from build123d import *

# Parameters (mm, degrees)
F1_DEPTH  = 6
F2_W      = 104
F2_H      = 80
F2_W_2    = 6
F3_DEPTH  = 6
F5_DEPTH  = 104
F7_DEPTH  = 200
F8_R      = 11.4401294272
F10_DEPTH = 200
F11_W     = 86
F11_H     = 24.3039056659
F12_DEPTH = 1
F13_W     = 32.8389904462
F13_H     = 60.4005604982
F14_DEPTH = 1


with BuildPart() as f1:
    # F0 (on Front) → F1 (new body)
    with BuildSketch(Plane.XZ):
        Polygon((-88, 80), (-80, 37.097658962), (-80, 80), align=None)
        Polygon((-80, 0), (0, 0), (0, 80), (-80, 80), (-80, 37.097658962), align=None)
    extrude(amount=F1_DEPTH)

    # F2 (on face) → F3 (join)
    with BuildSketch(Plane.YZ):
        with Locations((52, 40)):
            Rectangle(F2_W, F2_H)
        with Locations((-3, 40)):
            Rectangle(F2_W_2, F2_H)
    extrude(amount=F3_DEPTH)

    # F5 (add, through all): a face of the model
    f5_faces = [f1.faces().sort_by_distance(p)[0] for p in [
        (-41.1141866674, 0, 40.6711029977),
    ]]
    extrude(f5_faces, amount=F5_DEPTH)

    # F6 (on face) → F7 (cut)
    with BuildSketch(Plane.YZ.offset(6)):
        Polygon((104, 0), (49, 10.5), (-6, 0), align=None)
    extrude(amount=-F7_DEPTH, mode=Mode.SUBTRACT)

    # F8 (on face) → F10 (cut)
    with BuildSketch(Plane(origin=(0, 104, 0), x_dir=(-1, 0, 0), z_dir=(0, 1, 0))):
        with Locations((58.3457089961, 57.7158816159)):
            Circle(F8_R)
    extrude(amount=-F10_DEPTH, mode=Mode.SUBTRACT)

    # F11 (on face) → F12 (join)
    with BuildSketch(Plane(origin=(-70.6266357892, 0, -13.1697495438), x_dir=(0, -1, 0), z_dir=(-0.983055103, 0, -0.1833102957))):
        with Locations((-49, 72.5469328463)):
            Rectangle(F11_W, F11_H)
    extrude(amount=F12_DEPTH)

    # F13 (on face) → F14 (join)
    with BuildSketch(Plane(origin=(0, 104, 0), x_dir=(-1, 0, 0), z_dir=(0, 1, 0))):
        with Locations((20.5245364923, 30.2002802491)):
            Rectangle(F13_W, F13_H)
    extrude(amount=F14_DEPTH)


solid = f1.part
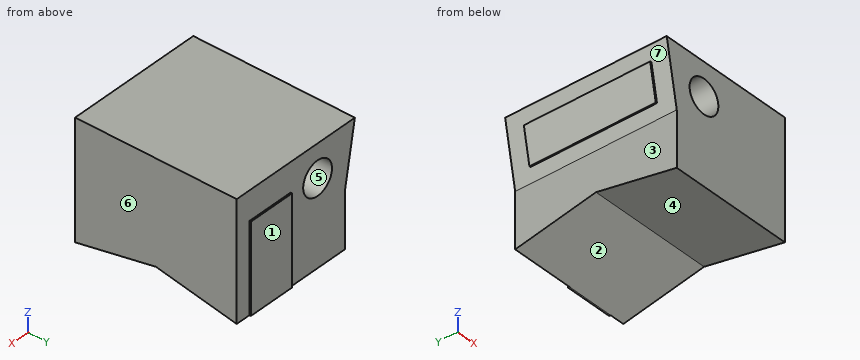
Geometry: final body of the model. Coordinates: model frame, mm. Face numbers are marked on the shaded views. A direction names the side the tool comes from. Give positions to 0.01 mm unless a question says otherwise; leave off trailing zeros. Loops run counter-clockwise (first coordinate to the right, second up) from the corner with the lowest first, then second, coordinate; pieces in that order, holes last. Notation, with made-up numbers: (-40, 30.5) -> (-9, 30.5) arc R22 ccw to (-9, 56.5) -> close; hole circle Ø5 at (-26.75, -20). An arc over 180 degrees is marked (long way). Put each result on its own line as item: value.
1. Pin query (flat end, axial travel): P1, Ø2.5, axis at x = -85.5, z = 59.5, coming from the +Y side; P2, Ø0.8, axis at y = 104.5, z = 15.5, coming from the -X side; P3, Ø6, axis at x = -66.5, z = 29.5, coming from the +Y side; P4, Ø13.5, axis at x = -58.35, z = 57.72, coming from the -Y side. Return the tip coordinate at first contact, or that it passes through.
Taken from the geometry:
P1: stops at y = 92
P2: stops at x = -36.94
P3: stops at y = 104
P4: passes through
2. Set-up query: the marked faces 1, 2 and 3. Return all of +Z, -Z, +X, -X, +Y, -Y with unobstructed straight access to the full face (end or side cutting, diameter ignored); none if empty.
Taken from the geometry:
face 1: +Z, -Z, +X, -X, +Y
face 2: -Z, +X, -X
face 3: -Z, -X, +Y, -Y
3. Cut plane A-A (z = 8.5). Return the cut outline in (x, y).
Taken from the geometry:
outline: (-80, -6) -> (6, -6) -> (6, 38.52) -> (-80, 38.52) -> close; (-80, 59.48) -> (6, 59.48) -> (6, 104) -> (-4.11, 104) -> (-4.11, 105) -> (-36.94, 105) -> (-36.94, 104) -> (-80, 104) -> close
4. Pull-direction query (Z, two-part tool) for the marked faces 4, 5, 6 and 7; classes: released by +Z, released by -Z, zero draft, split by the parting line, or undercut.
Taken from the geometry:
face 4: released by -Z
face 5: undercut
face 6: zero draft
face 7: undercut
5. Cut plane D-D (x = -28). Return the cut outline in (y, z).
Taken from the geometry:
outline: (-6, 0) -> (49, 10.5) -> (104, 0) -> (105, 0) -> (105, 60.4) -> (104, 60.4) -> (104, 80) -> (-6, 80) -> close
6. Cut plane B-B (z = 26.5). Return the cut outline in (x, y).
Taken from the geometry:
outline: (-80, -6) -> (6, -6) -> (6, 104) -> (-4.11, 104) -> (-4.11, 105) -> (-36.94, 105) -> (-36.94, 104) -> (-80, 104) -> close
7. Ray query, line 1 along Z through (x, y) = (-66, 66); line 2 along Y through (x, z) = (-46.5, 76); line 3 along Z through (x, y) = (-59, 17). Return the intervals inside material, ascending. Write a range as [from, to].
Taken from the geometry:
line 1: z = [7.25, 49.21], [66.22, 80]
line 2: y = [-6, 104]
line 3: z = [4.39, 46.29], [69.14, 80]
8. Cut plane C-C (y = 39). Return the cut outline in (x, z), plus the area to 3 significant figures.
Taken from the geometry:
outline: (-88, 80) -> (-86.15, 70.09) -> (-87.14, 69.91) -> (-82.68, 46.02) -> (-81.7, 46.2) -> (-80, 37.1) -> (-80, 8.59) -> (6, 8.59) -> (6, 80) -> close; hole circle Ø22.88 at (-58.35, 57.72)
area: 5,930 mm2
